Part model, mm, in its own coordinate system. A direction names the side the tool comes from. Round coordinates to 2 decimals unless told otherwise and drop trailing zeros. Answer as a JSON object with one key per item and string values.
```python
from build123d import *

# Parameters (mm, degrees)
SKETCH1_W                                           = 250
SKETCH1_H                                           = 250
SKETCH1_R                                           = 37
SKETCH1_R_2                                         = 26
BOSS_EXTRUDE1_DEPTH                                 = 10
M3_CLEARANCE_HOLE1_D                                = 3.4
CBORE_FOR_M6_HEX_SOCKET_HEAD_CAP_SCREW1_D           = 6.6
CBORE_FOR_M6_HEX_SOCKET_HEAD_CAP_SCREW1_CBORE_D     = 11
CBORE_FOR_M6_HEX_SOCKET_HEAD_CAP_SCREW1_CBORE_DEPTH = 6.4
F_2_5MM_CHAMFER1_SIZE                               = 2.5


with BuildPart() as part:
    # Sketch1 → Boss-Extrude1 (new body)
    # profile 1 of 2: a face of its own
    with BuildSketch(Plane(origin=(0, 0, 0), x_dir=(1, 0, 0), z_dir=(0, 1, 0))):
        Rectangle(SKETCH1_W, SKETCH1_H)
        Circle(SKETCH1_R, mode=Mode.SUBTRACT)
    # profile 2 of 2: a face of its own
    with BuildSketch(Plane(origin=(0, 0, 0), x_dir=(1, 0, 0), z_dir=(0, 1, 0))):
        Circle(SKETCH1_R)
        with Locations(Location((0, 0, 0), (0, 0, 270))):
            Circle(SKETCH1_R_2, mode=Mode.SUBTRACT)
    extrude(amount=BOSS_EXTRUDE1_DEPTH)

    # M3 Clearance Hole1 (through all)
    with Locations(Plane(origin=(0, 10, 0), x_dir=(1, 0, 0), z_dir=(0, 1, 0))):
        with Locations((0, 33), (28.578838325, 16.5), (28.578838325, -16.5), (0, -33), (-28.578838325, -16.5), (-28.578838325, 16.5)):
            Hole(M3_CLEARANCE_HOLE1_D / 2)

    # CBORE for M6 Hex Socket Head Cap Screw1 (through all)
    with Locations(Plane(origin=(0, 10, 0), x_dir=(1, 0, 0), z_dir=(0, 1, 0))):
        with Locations((-102.5, 102.5), (-34.16666667, 102.5), (34.16666666, 102.5), (102.5, 102.5), (102.49999999, 34.16666667), (102.49999999, -34.16666666), (102.5, -102.5), (34.16666666, -102.49999999), (-34.16666667, -102.49999999), (-102.5, -102.5), (-102.5, -34.16666666), (-102.5, 34.16666667)):
            CounterBoreHole(CBORE_FOR_M6_HEX_SOCKET_HEAD_CAP_SCREW1_D / 2, CBORE_FOR_M6_HEX_SOCKET_HEAD_CAP_SCREW1_CBORE_D / 2, CBORE_FOR_M6_HEX_SOCKET_HEAD_CAP_SCREW1_CBORE_DEPTH)

    # 2,5mm Chamfer1
    f_2_5mm_chamfer1_edges = [part.edges().sort_by_distance(p)[0] for p in [
        (125, 10, 0),
        (0, 10, -125),
        (-125, 10, 0),
        (0, 10, 125),
    ]]
    chamfer(f_2_5mm_chamfer1_edges, length=F_2_5MM_CHAMFER1_SIZE)


solid = part.part
```
Item 1: Probe L1, parallel to Z at x = -102.5, y = 7.25; L2, parallel to X at y = 2.2, z = 102.5; L3, parallel to X at y = 8.75, z = 102.5. List the from-to ranges inside material, lowest first. Write a range as from..to.
Taken from the geometry:
{"L1": "-125..-108, -97..-39.67, -28.67..28.67, 39.67..97, 108..125", "L2": "-125..-105.8, -99.2..-37.47, -30.87..30.87, 37.47..99.2, 105.8..125", "L3": "-123.75..-108, -97..-39.67, -28.67..28.67, 39.67..97, 108..123.75"}
Item 2: Two-plate mould, pull along Z, no slides. Class faces 3 (the flat face through (-2, 4, 125)), 4 (the flat face through (-29, 10, -2)), 5 (the flat face through (-99, 3.6, -34)): pulls with the +Z half, pulls with the -Z half, needs draft (parallel to the pull), parting line crosses it, or undercut.
Taken from the geometry:
{"face 3": "pulls with the +Z half", "face 4": "needs draft", "face 5": "undercut"}
Item 3: Drop a flat-ended pin along its axis: P1, Ø5.5, axis at x = -36.5, z = 102, coming from the +Y side. Give the stop position or say it passes through.
Taken from the geometry:
{"P1": "y = 3.6"}
Item 4: Cut at A-A (y = 5.25). State how many separate pieces and enclosed holes the cut face has, plus the area to 3 significant figures.
Taken from the geometry:
{"separate pieces": "1", "enclosed holes": "19", "area": "59,200 mm2"}
Item 5: Tool access for faces 1 (the flat face through (125, 4, 2)), 2 (the cylindrical face through (98.45, 6.84, 98.78)): list every direction of +Z, -Z, +X, -X, +Y, -Y with a clear straight run to the whole face (end or side of a thin tool).
Taken from the geometry:
{"face 1": "+Z, -Z, +X, +Y, -Y", "face 2": "+Y"}
